The model under review builds one solid part; all positions refer to its coordinate system, in mm. A direction names the side the tool comes from. Coordinates: 2 decimals unless noted, no trailing zeros. Loops run counter-clockwise (first coordinate to the right, second up) from the corner with the lowest first, then second, coordinate; pieces in that order, holes last. Notation, with made-up numbers: (31, 48) - (38, 48) arc R27 ccw to (38, 75) - close; hole circle Ø5 at (8.25, -12). An arc over 180 degrees is marked (long way). Use a Markdown table: item, result. Add a question column.
1) To check wall thickness, follow L1, parallel to Y at x = 25, z = -3.5 (1 decimal); L2, parallel to X at y = 43.5, z = -0.75; L3, parallel to Z at x = 63, y = 32. State the ranges of each line that lie inside material, in increasing order. Write a range as [from, to].
2) For faces 4 (the flat face through (61.7, 31.84, 0.78)), 5 (the flat face through (72, 19.05, -2)), 6 (the flat face through (17.7, -3.175, -3.2)), list the 3-axis set-ups (+Z, -Z, +X, -X, +Y, -Y) from which the entire face can be reached by the end or side of a thin tool; tool diameter is ignored.
3) Add section B-B, the plane y = 26. Give the boundary of the cut face in (x, z).
4) Clearance check with flat-ended pins moving along their axes: pin 1 (1.6 mm diameter, centred on y = 45, z = -2.5, fed in from +X); pin 2 (2 mm diameter, centred on x = 123.82, z = -2.38, fed in from +Y); pin 3 (4 mm diameter, centred on x = 102, z = -3.5, fed in from +Y); pin 4 (3.5 mm diameter, centred on y = -3.5, z = -2, fed in from +X). State where each tip first meets the part, or that it passes through.
5) The part is to be moulded in two halves that separate along X. For faces 1 (the cylindrical face through (21.08, -2.39, -2.68)), 2 (the flat face through (18, 42.776, -5)), 3 (the flat face through (35.83, 11.27, 0.78)), say which applies: pulls with the +X half, pulls with the -X half, needs draft (parallel to the pull), parting line crosses it, or undercut.
```python
from build123d import *

# Parameters (mm, degrees)
F1_DEPTH      = 1.5875
F3_DEPTH      = 4.7625
F4_W          = 6.35
F4_H          = 6.35
F4_W_2        = 4.7625
F4_H_2        = 4.7625
F5_DEPTH      = 3.175
F6_SIZE       = 1.8598642
F7_W          = 28.575
F7_H          = 3.175
F8_DEPTH      = 1.5875
F9_W          = 6.35
F9_H          = 1.5875
F10_DEPTH     = 6.35
F11_R         = 1.0922
F11_R_2       = 1.63322
F12_DEPTH     = 25.4
F13_SIZE      = 1.58749
F14_R         = 0.396875
F15_DEPTH     = 6.35
F16_R         = 1.63322
F17_DEPTH     = 1.5875
F18_W         = 141.7602359697
F18_H         = 50.7137336135
F19_DEPTH     = 7.9375
F20_W         = 1.5875
F20_H         = 3.175
F21_DEPTH     = 1.5875
F22_R         = 0.396875
F23_DEPTH     = 3.175
F24_T4_DEPTH  = 1.4175116858
F24_S5_R      = 0.396875
F24_T6_DEPTH  = 2
F24_T10_DEPTH = 1.4175116858
F24_S11_R     = 0.396875
F24_T12_DEPTH = 2
F24_T16_DEPTH = 2.8350233717
F24_S17_R     = 0.396875
F24_T18_DEPTH = 3


# Not quite as in the source:
# - a fillet or chamfer that OpenCascade refuses, or shapes differently, is made with other operations: its cross-section is extruded or revolved along the edge and cut away or added
# - a fillet or chamfer is up to 0.001 mm smaller than in the source, because OpenCascade refuses the exact size


with BuildPart() as f1:
    # F0 (on Top) → F1 (new body)
    with BuildSketch(Plane.XY):
        Polygon((-87.87765, 22.225), (-127, 22.225), (-127, 17.4625), (-48.7553, 17.4625), (-26.5303, -4.7625), (26.5303, -4.7625), (48.7553, 17.4625), (127, 17.4625), (127, 22.225), (87.87765, 22.225), (46.7826079092, 45.9512336135), (-46.7826079092, 45.9512336135), align=None)
        Polygon((-24.5576079092, 0), (-46.7826079092, 22.225), (-78.35265, 22.225), (-45.5064998802, 41.1887336135), (45.5064998802, 41.1887336135), (78.35265, 22.225), (46.7826079092, 22.225), (24.5576079092, 0), align=None, mode=Mode.SUBTRACT)
    extrude(amount=F1_DEPTH)

    # F2 (on face) → F3 (join)
    with BuildSketch(Plane(origin=(0, 0, 0), x_dir=(1, 0, 0), z_dir=(0, 0, -1))):
        Polygon((-48.7553, -17.4625), (-127, -17.4625), (-127, -19.05), (-93.376911314, -19.05), (-87.87765, -22.225), (-46.7826079092, -45.9512336135), (46.7826079092, -45.9512336135), (87.87765, -22.225), (93.376911314, -19.05), (127, -19.05), (127, -17.4625), (48.7553, -17.4625), (26.5303, 4.7625), (-26.5303, 4.7625), align=None)
        Polygon((-48.0977359697, -19.05), (-25.8727359697, 3.175), (-4.2897640303, 3.175), (-4.2897640303, 1.5875), (24.2852359697, 1.5875), (24.2852359697, 3.175), (25.8727359697, 3.175), (48.0977359697, -19.05), (90.201911314, -19.05), (46.3572385662, -44.3637336135), (24.2852359697, -44.3637336135), (24.2852359697, -42.7762336135), (-4.2897640303, -42.7762336135), (-4.2897640303, -44.3637336135), (-46.3572385662, -44.3637336135), (-90.201911314, -19.05), align=None, mode=Mode.SUBTRACT)
    extrude(amount=F3_DEPTH)

    # F4 (on face) → F5 (join, through all)
    with BuildSketch(Plane(origin=(0, 19.05, 0), x_dir=(-1, 0, 0), z_dir=(0, 1, 0))):
        with Locations((-53.5178, -1.5875)):
            Rectangle(F4_W, F4_H)
        with Locations((-123.825, -1.5875)):
            Rectangle(F4_W, F4_H)
        with Locations((124.61875, -2.38125)):
            Rectangle(F4_W_2, F4_H_2)
        with Locations((55.89905, -2.38125)):
            Rectangle(F4_W_2, F4_H_2)
    extrude(amount=F5_DEPTH)

    # F6
    f6_edges = [f1.edges().sort_by_distance(p)[0] for p in [
        (-127, 19.84375, -4.7625),
        (-122.2375, 20.6375, -4.7625),
        (-58.2803, 20.6375, -4.7625),
        (-53.5178, 20.6375, -4.7625),
        (50.3428, 20.6375, -4.7625),
        (56.6928, 20.6375, -4.7625),
        (120.65, 20.6375, -4.7625),
        (127, 19.84375, -4.7625),
    ]]
    chamfer(f6_edges, length=F6_SIZE)

    # F7 (on face) → F8 (join)
    with BuildSketch(Plane(origin=(0, 0, -4.7625), x_dir=(1, 0, 0), z_dir=(0, 0, -1))):
        with Locations((9.9977359697, 3.175)):
            Rectangle(F7_W, F7_H)
        with Locations((9.9977359697, -44.3637336135)):
            Rectangle(F7_W, F7_H)
    extrude(amount=F8_DEPTH)

    # F9 (on face) → F10 (cut, through all)
    with BuildSketch(Plane(origin=(0, 0, -6.35), x_dir=(1, 0, 0), z_dir=(0, 0, -1))):
        with Locations((19.5227359697, 3.96875)):
            Rectangle(F9_W, F9_H)
        with Locations((19.5227359697, -45.1574836135)):
            Rectangle(F9_W, F9_H)
    extrude(amount=-F10_DEPTH, mode=Mode.SUBTRACT)

    # F11 (on face) → F12 (cut, through all)
    with BuildSketch(Plane.XZ.offset(3.175)):
        with Locations((53.5178, -2.38125)):
            Circle(F11_R)
        with Locations((123.825, -2.38125)):
            Circle(F11_R)
        with Locations((-124.61875, -2.38125)):
            Circle(F11_R)
        with Locations((-55.89905, -2.38125)):
            Circle(F11_R)
        with Locations((19.5227359697, -3.175)):
            Circle(F11_R_2)
    extrude(amount=-F12_DEPTH, mode=Mode.SUBTRACT)

    # F13 (size 1.5875 in the source; OpenCascade refuses exactly that, so slightly less here)
    f13_edges = [f1.edges().sort_by_distance(p)[0] for p in [
        (-4.289764, -3.96875, -4.7625),
        (24.285236, -3.96875, -4.7625),
        (-4.289764, 45.157484, -4.7625),
        (24.285236, 45.157484, -4.7625),
    ]]
    chamfer(f13_edges, length=F13_SIZE)

    # F14 (on face) → F15 (cut, through all)
    with BuildSketch(Plane(origin=(0, 0, -6.35), x_dir=(1, 0, 0), z_dir=(0, 0, -1))):
        with Locations((22.6977359697, 3.175)):
            Circle(F14_R)
        with Locations((22.6977359697, -44.3637336135)):
            Circle(F14_R)
    extrude(amount=-F15_DEPTH, mode=Mode.SUBTRACT)

    # F16 (on face) → F17 (cut, through all)
    with BuildSketch(Plane(origin=(0, 44.3637336135, 0), x_dir=(-1, 0, 0), z_dir=(0, 1, 0))):
        with Locations((-19.5227359697, -3.175)):
            Circle(F16_R)
    extrude(amount=-F17_DEPTH, mode=Mode.SUBTRACT)

    # F18 (on face) → F19 (cut, through all)
    with BuildSketch(Plane(origin=(0, 0, -6.35), x_dir=(1, 0, 0), z_dir=(0, 0, -1))):
        with Locations((-56.1198820151, -20.5943668067)):
            Rectangle(F18_W, F18_H)
    extrude(amount=-F19_DEPTH, mode=Mode.SUBTRACT)

    # F20 (on face) → F21 (cut, through all)
    with BuildSketch(Plane.YZ.offset(16.3477359697)):
        with Locations((-3.96875, -4.7625)):
            Rectangle(F20_W, F20_H)
        with Locations((45.1574836135, -4.7625)):
            Rectangle(F20_W, F20_H)
    extrude(amount=-F21_DEPTH, mode=Mode.SUBTRACT)

    # F22 (on face) → F23 (cut, through all)
    with BuildSketch(Plane(origin=(0, 0, -3.175), x_dir=(1, 0, 0), z_dir=(0, 0, -1))):
        with Locations((16.3477359697, -44.3637336135)):
            Circle(F22_R)
        with Locations((16.3477359697, 3.175)):
            Circle(F22_R)
    extrude(amount=-F23_DEPTH, mode=Mode.SUBTRACT)

    # F24: chamfer of 0.396875 on 3 edges, made by hand


with BuildPart() as f24_tool2:
    # F24_s3 → F24_t4 (new body)
    with BuildSketch(Plane.YZ.offset(17.7652476556)):
        Polygon((-2.778125, -3.175), (-3.175, -3.571875), (-3.175, -3.175), align=None)
    extrude(amount=-F24_T4_DEPTH)

    # F24_s5 → F24_t6 (intersect, symmetric)
    with BuildSketch(Plane.XY.offset(-3.4)):
        with Locations((16.3477359697, -3.175)):
            Circle(F24_S5_R)
    extrude(amount=F24_T6_DEPTH, both=True, mode=Mode.INTERSECT)


with BuildPart() as f1_1:
    add(f1.part)

    # F24_t1: cut F24_tool2
    add(f24_tool2.part, mode=Mode.SUBTRACT)


with BuildPart() as f24_tool8:
    # F24_s9 → F24_t10 (new body)
    with BuildSketch(Plane.YZ.offset(16.3477359697)):
        Polygon((-2.778125, -3.175), (-3.175, -3.571875), (-3.175, -3.175), align=None)
    extrude(amount=-F24_T10_DEPTH)

    # F24_s11 → F24_t12 (intersect, symmetric)
    with BuildSketch(Plane.XY.offset(-3.4)):
        with Locations((16.3477359697, -3.175)):
            Circle(F24_S11_R)
    extrude(amount=F24_T12_DEPTH, both=True, mode=Mode.INTERSECT)


with BuildPart() as f1_2:
    add(f1_1.part)

    # F24_t7: cut F24_tool8
    add(f24_tool8.part, mode=Mode.SUBTRACT)


with BuildPart() as f24_tool14:
    # F24_s15 → F24_t16 (new body)
    with BuildSketch(Plane.YZ.offset(14.9302242839)):
        Polygon((44.3637336135, -3.571875), (43.9668586135, -3.175), (44.3637336135, -3.175), align=None)
    extrude(amount=F24_T16_DEPTH)

    # F24_s17 → F24_t18 (intersect, symmetric)
    with BuildSketch(Plane.XY.offset(-3.4)):
        with Locations((16.3477359697, 44.3637336135)):
            Circle(F24_S17_R)
    extrude(amount=F24_T18_DEPTH, both=True, mode=Mode.INTERSECT)


with BuildPart() as f1_3:
    add(f1_2.part)

    # F24_t13: cut F24_tool14
    add(f24_tool14.part, mode=Mode.SUBTRACT)


solid = f1_3.part
```
From the geometry:
| question | item | result |
|---|---|---|
| 1 | L1 | y = [-4.8, -3.2], [44.4, 46] |
| 1 | L2 | x = [14.76, 24.29], [47.85, 51.03] |
| 1 | L3 | z = [0, 1.59] |
| 2 | face 4 | +Z, -Z, -X |
| 2 | face 5 | -Z |
| 2 | face 6 | -Z, -Y |
| 3 | outline | (71.81, 0) - (78.16, 0) - (78.16, -4.76) - (81.34, -4.76) - (81.34, 1.59) - (71.81, 1.59) - close |
| 4 | pin 1 | stops at x = 49.82 |
| 4 | pin 2 | passes through |
| 4 | pin 3 | stops at y = 19.05 |
| 4 | pin 4 | stops at x = 29.54 |
| 5 | face 1 | undercut |
| 5 | face 2 | needs draft |
| 5 | face 3 | pulls with the -X half |
